Autodesk Inventor part; units mm, degrees
ref_plane "YZ Plane" through (0, 0, 0) normal (1, 0, 0) x (0, 1, 0)
ref_plane "XZ Plane" through (0, 0, 0) normal (0, 1, 0) x (-1, 0, 0)
ref_plane "XY Plane" through (0, 0, 0) normal (0, 0, 1) x (1, 0, 0)
sketch "Esboço1" plane through (0, 0, 0) normal (0, 0, 1) x (1, 0, 0)
  line L0 (-60, -60) -> (60, -60)
  line L1 (60, -60) -> (60, 60)
  line L2 (60, 60) -> (-60, 60)
  line L3 (-60, 60) -> (-60, -60)
  line L4 (-60, -60) -> (60, 60) construction
  line L5 (60, -60) -> (-60, 60) construction
  point P0 (0, 0)
  dimension "d0" = 120
  dimension "d1" = 120
extrude "Extrusão1" add sketch "Esboço1" along normal blind 3
sketch "Esboço2" plane through (-60, 60, 0) normal (0, 1, 0) x (1, 0, 0)
  line L0 (120, -3) -> (0, -3)
  line L1 (120, 0) -> (0, 0)
  line L2 (0, -3) -> (15.1, -3)
  line L3 (15.1, -3) -> (15.1, 0)
  line L4 (15.1, 0) -> (0, 0)
  line L5 (0, 0) -> (0, -3)
  line L6 (-0.1, 0) -> (-0.1, -3)
  line L7 (29.9, 0) -> (29.9, -3)
  line L8 (45.1, 0) -> (30, 0)
  line L9 (30, -3) -> (45.1, -3)
  line L10 (45.1, -3) -> (45.1, 0)
  line L11 (59.9, 0) -> (59.9, -3)
  line L12 (75.1, 0) -> (60, 0)
  line L13 (60, -3) -> (75.1, -3)
  line L14 (75.1, -3) -> (75.1, 0)
  line L15 (89.9, 0) -> (89.9, -3)
  line L16 (105.1, 0) -> (90, 0)
  line L17 (90, -3) -> (105.1, -3)
  line L18 (105.1, -3) -> (105.1, 0)
  point P0 (89.9, 0)
  point P1 (59.9, 0)
  point P2 (29.9, 0)
  dimension "d4" = 15.1
  dimension "d57" = 30
  dimension "d63" = 0.1
extrude "Extrusão2" cut sketch "Esboço2" against normal blind 3 contours L0 L15 L1 L18 | L0 L11 L1 L14 | L0 L7 L1 L10 | L0 L5 L1 L3
sketch "Esboço3" plane through (-60, -60, 0) normal (0, -1, 0) x (1, 0, 0)
  line L0 (0, 0) -> (120, 0)
  line L1 (0, 3) -> (15.1, 3)
  line L2 (15.1, 3) -> (15.1, 0)
  line L3 (15.1, 0) -> (0, 0)
  line L4 (0, 0) -> (0, 3)
  line L5 (-0.1, 0) -> (-0.1, 3)
  line L6 (-0.1, 0) -> (15.1, 0)
  line L7 (15.1, 0) -> (15.1, 3)
  line L8 (15.1, 3) -> (-0.1, 3)
  line L9 (-0.1, 3) -> (-0.1, 0)
  line L10 (29.9, 0) -> (29.9, 3)
  line L11 (45.1, 0) -> (30, 0)
  line L12 (30, 3) -> (45.1, 3)
  line L13 (45.1, 3) -> (45.1, 0)
  line L14 (59.9, 0) -> (59.9, 3)
  line L15 (75.1, 0) -> (60, 0)
  line L16 (60, 3) -> (75.1, 3)
  line L17 (75.1, 3) -> (75.1, 0)
  line L18 (89.9, 0) -> (89.9, 3)
  line L19 (105.1, 0) -> (90, 0)
  line L20 (90, 3) -> (105.1, 3)
  line L21 (105.1, 3) -> (105.1, 0)
  line L22 (0, 0) -> (0, 3)
  line L23 (0, 3) -> (120, 3)
  line L24 (120, 3) -> (120, 0)
  line L25 (120, 0) -> (0, 0)
  point P0 (-0.1, 1.5)
  point P1 (29.9, 1.5)
  point P2 (59.9, 1.5)
  point P3 (89.9, 1.5)
  point P4 (105.1, 0)
  point P5 (89.9, 0)
  point P6 (75.1, 0)
  point P7 (59.9, 0)
  point P8 (45.1, 0)
  point P9 (29.9, 0)
  dimension "d14" = 15.1
  dimension "d47" = 15.2
  dimension "d50" = 30
  dimension "d64" = 0.1
extrude "Extrusão3" cut sketch "Esboço3" against normal blind 3 contours L4 L1 L2 L0 | L10 L23 L12 L13 L0 | L14 L23 L16 L17 L0 | L18 L23 L20 L21 L0
sketch "Esboço5" plane through (60, -60, 0) normal (1, 0, 0) x (0, 0, -1)
  line L0 (0, 3) -> (-3, 3)
  line L1 (-3, 3) -> (0, 3)
  line L2 (0, 3) -> (0, 18.1)
  line L3 (0, 18.1) -> (-3, 18.1)
  line L4 (-3, 18.1) -> (-3, 3)
  line L5 (0, 0) -> (-3, 0)
  line L6 (-3, 0) -> (-3, 120)
  line L7 (-3, 120) -> (0, 120)
  line L8 (0, 120) -> (0, 0)
  line L9 (0, 0) -> (-3, 0)
  line L10 (-3, 0) -> (-3, 120)
  line L11 (-3, 120) -> (0, 120)
  line L12 (0, 120) -> (0, 0)
  line L13 (-3, 3.1) -> (0, 3.1)
  line L14 (-3, 33.1) -> (0, 33.1)
  line L15 (0, 48.1) -> (-3, 48.1)
  line L16 (-3, 63.1) -> (0, 63.1)
  line L17 (0, 78.1) -> (-3, 78.1)
  line L18 (-3, 93.1) -> (0, 93.1)
  line L19 (0, 108.1) -> (-3, 108.1)
  line L20 (-3, 123.1) -> (0, 123.1)
  line L21 (0, 138.1) -> (-3, 138.1)
  line L22 (-3, 153.1) -> (0, 153.1)
  line L23 (0, 168.1) -> (-3, 168.1)
  line L24 (-3, 183.1) -> (0, 183.1)
  line L25 (0, 198.1) -> (-3, 198.1)
  line L26 (-3, 213.1) -> (0, 213.1)
  line L27 (0, 228.1) -> (-3, 228.1)
  line L28 (-3, 243.1) -> (0, 243.1)
  line L29 (0, 258.1) -> (-3, 258.1)
  line L30 (-3, 273.1) -> (0, 273.1)
  line L31 (0, 288.1) -> (-3, 288.1)
  line L32 (-3, 117.1) -> (0, 117.1)
  point P0 (-1.5, 3)
  point P1 (-3, 3.1)
  point P2 (-1.5, 120)
  dimension "d35" = 3
  dimension "d36" = 15.1
  dimension "d65" = 0.1
  dimension "d68" = 30
  dimension "d73" = 2.9
extrude "Extrusão5" add sketch "Esboço5" along normal blind 3 contours L8 L5 L6 L0 | L0 L4 L13 L2 | L13 L4 L3 L2 | L14 L6 L15 L8 | L16 L6 L17 L8 | L18 L6 L19 L8 | L32 L6 L7 L8
sketch "Esboço6" plane through (0, 0, 3) normal (0, 0, 1) x (1, 0, 0)
  line L0 (-54.8, -53.9) -> (-57, -53.9)
  line L1 (-57, -53.9) -> (-57, 53.9)
  line L2 (-57, 53.9) -> (-54.8, 53.9)
  line L3 (-54.8, 53.9) -> (-54.8, -53.9)
  line L4 (-54.8, -53.9) -> (-57, 53.9) construction
  line L5 (-57, -53.9) -> (-54.8, 53.9) construction
  line L6 (-44.9, 57) -> (-60, 57)
  line L7 (-60, 57) -> (-60, -57)
  point P0 (0, 0)
  point P1 (-55.9, 0)
  dimension "d74" = 3.1
  dimension "d75" = 3
  dimension "d76" = 2.2
extrude "Extrusão6" cut sketch "Esboço6" against normal up to surface (3 mm away)
properties part number "Base"
Verification items for the finished model (mm, model axes). A direction names the side the tool comes from. Round coordinates to 2 decimals unless told otherwise and drop trailing zeros. Order: outer loops, then holes, each group sorted by start corner. A loop starts at its lowest first (then second) coordinate and runs counter-clockwise, first axis right, second up. Notation, with made-up numbers: (56, -15) -> (94, -15) arc R29 ccw to (94, 22) -> close; hole circle Ø7 at (41, -2.5). An arc over 180 degrees is marked (long way). Put each result on its own line as item: value. Start each with the question number.
(1) Material ranges on line 1 along X through (y, z) = (-1.5, 1.15); line 2 along X through (y, z) = (-14.5, 2.8); line 3 along Y through (x, z) = (-15, 0.4), recorded low to high.
(2) Tool access check on faces 4 (the face through (29.9, 59, 1)), 5 (the face through (60, -35, 1)), 6 (the face through (29.9, -59, 1)), 7 (the face through (-38, -60, 1)), 8 (the face through (23, 60, 1)). Record the directions out of +Z, -Z, +X, -X, +Y, -Y that give a thin tool (end or side, any length) a straight path to the whole face; none if there is none.
(3) Section check A-A (y = -6.5). Enter the section's corners in (x, z).
(4) Section check B-B (y = -49). Enter the section's corners in (x, z).
(5) Draft check along Y on faces 1 (the face through (15.1, 59, 2)), 2 (the face through (7, 57, 1)), 3 (the face through (60, 25, 1)). Enter one of: +Y half, -Y half, draft (parallel to the pull), parting line (faces both ways), or undercut.
(6) Depth check by flat-ended pin: pin 1 Ø0.9 at (y, z) = (58, 1) entering from -X; pin 2 Ø5 at (x, y) = (46.5, -10) entering from -Z; pin 3 Ø0.9 at (x, z) = (-51.5, 1.5) entering from +Y; pin 4 Ø1.5 at (y, z) = (52.5, 2) entering from +X. Enter the tip coordinate at first touch or a pass-through.
Completed:
1. line 1: x = -60 to -57, -54.8 to 60
1. line 2: x = -60 to -57, -54.8 to 63
1. line 3: y = -57 to 57
2. face 4: +Z, -Z, +Y
2. face 5: +Z, -Z, +X
2. face 6: +Z, -Z, -Y
2. face 7: +Z, -Z, +X, -X, -Y
2. face 8: +Z, -Z, +X, -X, +Y
3. outline: (-60, 0) -> (-57, 0) -> (-57, 3) -> (-60, 3) -> close; (-54.8, 0) -> (60, 0) -> (60, 3) -> (-54.8, 3) -> close
4. outline: (-60, 0) -> (-57, 0) -> (-57, 3) -> (-60, 3) -> close; (-54.8, 0) -> (63, 0) -> (63, 3) -> (-54.8, 3) -> close
5. face 1: draft
5. face 2: +Y half
5. face 3: undercut
6. pin 1: stops at x = -44.9
6. pin 2: stops at z = 0
6. pin 3: stops at y = 57
6. pin 4: stops at x = 60
